from build123d import *

# Parameters (mm, degrees)
SKETCH1_R           = 13.335
FEATUREA_DEPTH      = 38.1
SKETCH2_W           = 26.67
SKETCH2_H           = 38.1
FEATUREB_DEPTH      = 1.778
FEATUREC_DEPTH      = 11.43
SKETCH4_W           = 1.27
SKETCH4_H           = 38.1
FEATURED_DEPTH      = 38.1
SKETCH7_W           = 13.97
SKETCH7_H           = 38.1
BOSS_EXTRUDE5_DEPTH = 29.21


with BuildPart() as part:
    # Sketch1 → FeatureA (new body)
    with BuildSketch(Plane.XY):
        Circle(SKETCH1_R)
    extrude(amount=-FEATUREA_DEPTH)

    # Sketch2 → FeatureB (add)
    with BuildSketch(Plane(origin=(0, 0, -38.1), x_dir=(-1, 0, 0), z_dir=(0, 0, -1))):
        with Locations((0, 19.05)):
            Rectangle(SKETCH2_W, SKETCH2_H)
    extrude(amount=-FEATUREB_DEPTH)

    # Sketch3 → FeatureC (add)
    with BuildSketch(Plane(origin=(0, 38.1, 0), x_dir=(1, 0, 0), z_dir=(0, 1, 0))):
        Polygon((0, 38.1), (-33.02, 38.1), (-33.02, 0), (33.02, 0), (33.02, 38.1), align=None)
    extrude(amount=FEATUREC_DEPTH)

    # Sketch4 → FeatureD (add)
    with BuildSketch(Plane(origin=(0, 49.53, 0), x_dir=(1, 0, 0), z_dir=(0, 1, 0))):
        with Locations((32.385, 19.05)):
            Rectangle(SKETCH4_W, SKETCH4_H)
        with Locations((-32.385, 19.05)):
            Rectangle(SKETCH4_W, SKETCH4_H)
    extrude(amount=FEATURED_DEPTH)

    # Sketch7 → Boss-Extrude5 (add)
    with BuildSketch(Plane(origin=(0, 87.63, 0), x_dir=(1, 0, 0), z_dir=(0, 1, 0))):
        with Locations((26.035, 19.05)):
            Rectangle(SKETCH7_W, SKETCH7_H)
        with Locations((-26.035, 19.05)):
            Rectangle(SKETCH7_W, SKETCH7_H)
    extrude(amount=BOSS_EXTRUDE5_DEPTH)


solid = part.part
Here's how the part is built. I have some questions about the finished solid (model axes, mm). A direction names the side the tool comes from. Coordinates: 2 decimals unless noted, no trailing zeros. Write each loop counter-clockwise with the first axis right and the second up, starting at its lowest first coordinate (ties: lowest second). Pieces come first, ordered by that corner, then holes.
1) If we section it at B-B (x = 20.5): List the corners of the cut face in (y, z) for me, plus the area to 3 significant figures.
Filled in:
outline: (38.1, -38.1) - (49.53, -38.1) - (49.53, 0) - (38.1, 0) - close; (87.63, -38.1) - (116.84, -38.1) - (116.84, 0) - (87.63, 0) - close
area: 1,550 mm2
2) If we section it at A-A (z = -30.5): List the corners of the cut face in (x, y) for me (3 decimals), plus the area to 3 significant figures.
Filled in:
outline: (-33.02, 38.1) - (33.02, 38.1) - (33.02, 116.84) - (19.05, 116.84) - (19.05, 87.63) - (31.75, 87.63) - (31.75, 49.53) - (-31.75, 49.53) - (-31.75, 87.63) - (-19.05, 87.63) - (-19.05, 116.84) - (-33.02, 116.84) - close; circle Ø26.67 at (0, 0)
area: 2,230 mm2
3) If we section it at C-C (y = 60): List the corners of the cut face in (x, z) for me, plus the area to 3 significant figures.
Filled in:
outline: (-33.02, -38.1) - (-31.75, -38.1) - (-31.75, 0) - (-33.02, 0) - close; (31.75, -38.1) - (33.02, -38.1) - (33.02, 0) - (31.75, 0) - close
area: 96.8 mm2
4) Which directions (+Z, -Z, +X, -X, +Y, -Y) give clear straight access to the entire face, cutting with the end or side of a thin tool? Please do faces 1 (the face through (-1.74, 13.22, -18.78)), 2 (the face through (-31.75, 68, -19)), 3 (the face through (-19.05, 102, -19)).
Filled in:
face 1: +Z
face 2: +Z, -Z
face 3: +Z, -Z, +Y
5) If I drill on line 1 (X direction, y = 111.5, z = -34.5); line 2 (Z direction, x = 9.5, y = 18.5); line 3 (Y direction, x = -7.5, z = -6), over which ranges is the centre line in solid material (lowest first)?
Filled in:
line 1: x = -33.02 to -19.05, 19.05 to 33.02
line 2: z = -38.1 to -36.32
line 3: y = -11.03 to 11.03, 38.1 to 49.53
6) Thinking about a two-plate mould opening in X: for faces 4 (the face through (-26, 116.84, -19)), 5 (the face through (-25, 87.63, -19)), 6 (the face through (33.02, 77, -19)), 7 (the face through (31.75, 68, -19)), which applies, +X half, -X half, draft (parallel to the pull), parting line (faces both ways), or undercut?
Filled in:
face 4: draft
face 5: undercut
face 6: +X half
face 7: undercut
7) I'm going to push flat-ended pins straight in: pin 1 (21.5 mm diameter, centred on x = 1.5, y = 25, fed in from +Z); pin 2 (6 mm diameter, centred on x = -1, z = -10.5, fed in from +Y); pin 3 (1 mm diameter, centred on x = 7.5, z = -28, fed in from -Y). Where does each tip first touch, or does it pass through?
Filled in:
pin 1: stops at z = -36.32
pin 2: stops at y = 49.53
pin 3: stops at y = -11.35
8) If we section it at D-D (x = 0): List the corners of the cut face in (y, z) for me (3 decimals).
Filled in:
outline: (-13.335, -38.1) - (49.53, -38.1) - (49.53, 0) - (38.1, 0) - (38.1, -36.322) - (13.335, -36.322) - (13.335, 0) - (-13.335, 0) - close
